Read the model definition and answer for the solid it produces. Units are mm, in the model's axes. A direction names the side the tool comes from. Give positions to 0.01 mm unless a question says otherwise; leave off trailing zeros. One line per item, written item: value.
from build123d import *

# Parameters (mm, degrees)
F0_W     = 107
F0_H     = 157
F1_DEPTH = 5
F2_R     = 1.475
F3_DEPTH = 5
F4_R     = 1.475
F5_DEPTH = 5
F6_W     = 20
F6_H     = 2.5
F7_DEPTH = 20


with BuildPart() as f1:
    # F0 (on Top) → F1 (new body)
    with BuildSketch(Plane.XY):
        Rectangle(F0_W, F0_H)
    extrude(amount=F1_DEPTH)

    # F2 (on face) → F3 (cut)
    with BuildSketch(Plane.YZ.offset(53.5)):
        with Locations((-76, 2.5)):
            Circle(F2_R)
        with Locations((-50.6667, 2.5)):
            Circle(F2_R)
        with Locations((-25.3334, 2.5)):
            Circle(F2_R)
        with Locations((-0.0001, 2.5)):
            Circle(F2_R)
        with Locations((25.3332, 2.5)):
            Circle(F2_R)
        with Locations((50.6665, 2.5)):
            Circle(F2_R)
        with Locations((75.9998, 2.5)):
            Circle(F2_R)
    extrude(amount=-F3_DEPTH, mode=Mode.SUBTRACT)

    # F4 (on face) → F5 (cut)
    with BuildSketch(Plane(origin=(-53.5, 0, 0), x_dir=(0, -1, 0), z_dir=(-1, 0, 0))):
        with Locations((-76, 2.5)):
            Circle(F4_R)
        with Locations((-50.6667, 2.5)):
            Circle(F4_R)
        with Locations((-25.3334, 2.5)):
            Circle(F4_R)
        with Locations((-0.0001, 2.5)):
            Circle(F4_R)
        with Locations((25.3332, 2.5)):
            Circle(F4_R)
        with Locations((50.6665, 2.5)):
            Circle(F4_R)
        with Locations((75.9998, 2.5)):
            Circle(F4_R)
    extrude(amount=-F5_DEPTH, mode=Mode.SUBTRACT)

    # F6 (on face) → F7 (cut)
    with BuildSketch(Plane.XZ.offset(78.5)):
        with Locations((0, 2.5)):
            Rectangle(F6_W, F6_H)
    extrude(amount=-F7_DEPTH, mode=Mode.SUBTRACT)


solid = f1.part
1) Each of these flat-tipped pins is pushed along its axis until it touches: pin 1 Ø1.8 at (y, z) = (-76, 2.5) entering from -X; pin 2 Ø6 at (x, y) = (-27, -22) entering from -Z; pin 3 Ø2.5 at (y, z) = (-25.33, 2.5) entering from +X. Where does it stop, or does it pass through?
Reported:
pin 1: stops at x = -48.5
pin 2: stops at z = 0
pin 3: stops at x = 48.5
2) Determine the mould class of faces 1 (the face through (0, -69, 3.75)), 2 (the face through (51.035, 24.163, 1.602)), 3 (the face through (-1, 78.5, 2)) for opening direction Y: +Y half, -Y half, draft (parallel to the pull), parting line (faces both ways), or undercut.
Reported:
face 1: draft
face 2: undercut
face 3: +Y half
3) Consider probe 1 along X at (y, z) = (-67.5, 3.5); probe 2 along X at (y, z) = (-0.5, 2.2). Determine where each line is inside the solid, lowest interval first.
Reported:
probe 1: x = -53.5 to -10, 10 to 53.5
probe 2: x = -48.5 to 48.5
4) Which of the six approach directions +Z, -Z, +X, -X, +Y, -Y give full straight-line access (tool end or side, diameter ignored) to faces 4 (the face through (-48.5, 25, 3)), 5 (the face through (51.035, 49.193, 2.565))?
Reported:
face 4: -X
face 5: +X
